Can you work these out from the model? Positions are in its coordinate system, mm. A direction names the side the tool comes from. Give positions to 0.01 mm unless a question says otherwise; leave off trailing zeros. Write each loop counter-clockwise with the first axis right and the second up, starting at its lowest first coordinate (ties: lowest second). Pieces come first, ordered by that corner, then holes.
1. If I drill on probe 1 along Y at (x, z) = (0, 6.75) (3 decimals); probe 2 along X at (y, z) = (7, 11.25); probe 3 along Y at (x, z) = (-9, 9.5), over which ranges is the centre line in solid material (lowest first)?
2. On a 3-axis mill with a long thin cutter (end or side, diameter ignored), from which of +Z, -Z, +X, -X, +Y, -Y can I reach the whole of each face in a straight line? I mean faces 4 (the cylindrical face through (-2.38, -10.74, 8.59)), 5 (the flat face through (11.4, 0.4, 15)). Say none if no direction works.
3. Suppose I cut it at C-C (z = 12.75). Please give me the cut outline in (x, y) (3 decimals), and give its area (3 significant figures).
4. Suppose I cut it at A-A (x = 0). Please give me the cut outline in (y, z).
5. Thinking about a two-plate mould opening in Y: for faces 1 (the flat face through (7.2, 2.6, 2)), 2 (the flat face through (5, 6, 0)), 3 (the conical face through (-5.512, -24.823, 4.272)), which applies, pulls with the +Y half, pulls with the -Y half, needs draft (parallel to the pull), parting line crosses it, or undercut?
6. Suppose I cut it at B-B (z = 8). Please give me the cut outline in (x, y).
7. I'm going to push flat-ended pins straight in: pin 1 (3 mm diameter, centred on x = -18, z = 8, fed in from +Y); pin 2 (1 mm diameter, centred on x = -21, y = -7, fed in from -Z); pin 3 (8 mm diameter, centred on x = 0, z = 12, fed in from +Y); pin 4 (4 mm diameter, centred on y = -5, z = 9, fed in from +X). Where does each tip first touch, or does it pass through?
```python
from build123d import *

# Parameters (mm, degrees)
F0_R     = 25
F2_R     = 26.5
F4_R     = 11
F5_DEPTH = 13
F6_R     = 7.5
F7_DEPTH = 25


with BuildPart() as f3:
    # F0 (on Top) → F3 section 0
    with BuildSketch(Plane.XY):
        Circle(F0_R)
    # F2 (on offset) → F3 section 1
    with BuildSketch(Plane.XY.offset(15)):
        Circle(F2_R)
    loft()

    # F4 (on face) → F5 (cut)
    with BuildSketch(Plane.XY.offset(15)):
        Circle(F4_R)
    extrude(amount=-F5_DEPTH, mode=Mode.SUBTRACT)

    # F6 (on face) → F7 (cut)
    with BuildSketch(Plane.XY.offset(2)):
        Circle(F6_R)
    extrude(amount=-F7_DEPTH, mode=Mode.SUBTRACT)


solid = f3.part
```
Checks:
1. probe 1: y = -25.675 to -11, 11 to 25.675
1. probe 2: x = -25.17 to -8.49, 8.49 to 25.17
1. probe 3: y = -24.34 to -6.32, 6.32 to 24.34
2. face 4: +Z
2. face 5: +Z, +X, -X, +Y, -Y
3. outline: circle Ø52.55 at (0, 0); hole circle Ø22 at (0, 0)
3. area: 1,790 mm2
4. outline: (-26.5, 15) - (-25, 0) - (-7.5, 0) - (-7.5, 2) - (-11, 2) - (-11, 15) - close; (7.5, 0) - (25, 0) - (26.5, 15) - (11, 15) - (11, 2) - (7.5, 2) - close
5. face 1: undercut
5. face 2: needs draft
5. face 3: parting line crosses it
6. outline: circle Ø51.6 at (0, 0); hole circle Ø22 at (0, 0)
7. pin 1: stops at y = 19.85
7. pin 2: stops at z = 0
7. pin 3: stops at y = 26.5
7. pin 4: stops at x = 25.8
